Geometry: final body of the model. Coordinates: model frame, mm. Face numbers are marked on the shaded views. A direction names the side the tool comes from. Give positions to 0.01 mm unless a question says otherwise; leave off trailing zeros. Write each loop counter-clockwise with the first axis right and the second up, starting at its lowest first coordinate (ties: lowest second). Pieces come first, ordered by that corner, then holes.
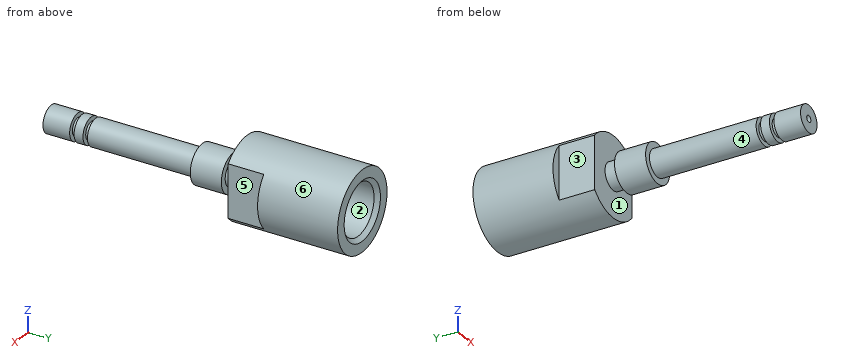
```python
from build123d import *

# Parameters (mm, degrees)
SKETCH17_R                    = 1.5
CUT_EXTRUDE1_DEPTH            = 65
G1_4_TAPPED_HOLE1_D           = 11.445
G1_4_TAPPED_HOLE1_DEPTH       = 22
G1_4_TAPPED_HOLE1_CSINK_D     = 13.207
G1_4_TAPPED_HOLE1_CSINK_ANGLE = 90
G1_4_TAPPED_HOLE1_TIP         = 3.438424892
SKETCH18_W                    = 13.595594723
SKETCH18_H                    = 16.071338344
CUT_EXTRUDE2_DEPTH            = 8


with BuildPart() as part:
    # Sketch1 → Revolve1 (revolve)
    with BuildSketch(Plane.XY):
        Polygon((-0.75, 0), (-0.75, 70), (-9, 70), (-9, 44), (-3, 44), (-3, 41), (-4.396039606, 41), (-4.396039606, 34), (-3, 34), (-3, 10), (-2, 10), (-2, 9), (-3, 9), (-3, 7), (-2, 7), (-2, 6), (-3, 6), (-3, 0), align=None)
    revolve(axis=Axis((0, 0, 0), (0, 1, 0)))

    # Sketch17 → Cut-Extrude1 (cut)
    with BuildSketch(Plane(origin=(0, 70, 0), x_dir=(1, 0, 0), z_dir=(0, 1, 0))):
        Circle(SKETCH17_R)
    extrude(amount=-CUT_EXTRUDE1_DEPTH, mode=Mode.SUBTRACT)

    # G1/4 Tapped Hole1
    with Locations(Plane(origin=(0, 70, 0), x_dir=(1, 0, 0), z_dir=(0, 1, 0))):
        with Locations((0, 0)):
            CounterSinkHole(G1_4_TAPPED_HOLE1_D / 2, G1_4_TAPPED_HOLE1_CSINK_D / 2, depth=G1_4_TAPPED_HOLE1_DEPTH, counter_sink_angle=G1_4_TAPPED_HOLE1_CSINK_ANGLE)
            with Locations((0, 0, -(G1_4_TAPPED_HOLE1_DEPTH + G1_4_TAPPED_HOLE1_TIP / 2))):  # 118° drill point
                Cone(0, G1_4_TAPPED_HOLE1_D / 2, G1_4_TAPPED_HOLE1_TIP, mode=Mode.SUBTRACT)

    # Sketch18 → Cut-Extrude2 (cut)
    with BuildSketch(Plane.XZ.offset(-44)):
        with Locations((-13.547797362, 0)):
            Rectangle(SKETCH18_W, SKETCH18_H)
        with Locations((13.547797362, 0)):
            Rectangle(SKETCH18_W, SKETCH18_H)
    extrude(amount=-CUT_EXTRUDE2_DEPTH, mode=Mode.SUBTRACT)


solid = part.part
```
Item 1: Line query: L1, parallel to Z at x = 0, y = 58; L2, parallel to Z at x = 0, y = 22.5; L3, parallel to Y at x = 7.25, z = -2.75. Output: solid intervals per line, ascending.
Found:
L1: z = -9 to -5.72, 5.72 to 9
L2: z = -3 to -1.5, 1.5 to 3
L3: y = 52 to 70
Item 2: Section A-A, the plane y = 40. Return the cut outline in (x, z).
Found:
outline: circle Ø8.79 at (0, 0); hole circle Ø3 at (0, 0)
Item 3: Section B-B, the plane x = 7.5. Return the cut outline in (y, z).
Found:
outline: (52, -4.97) - (70, -4.97) - (70, 4.97) - (52, 4.97) - close
Item 4: Pin query (flat end, axial travel): pin 1 Ø5 at (x, z) = (-0.5, -0.5) entering from -Y; pin 2 Ø3 at (x, z) = (0.5, 1) entering from +Y; pin 3 Ø6.5 at (y, z) = (46.5, -2) entering from +X; pin 4 Ø1 at (x, z) = (1, -2.5) entering from +Y. Return the tip coordinate at first contact, or that it passes through.
Found:
pin 1: stops at y = 0
pin 2: stops at y = 46.13
pin 3: stops at x = 6.75
pin 4: stops at y = 46.48
Item 5: Reachability of the marked faces 4, 5 and 6 from +Z, -Z, +X, -X, +Y, -Y: full face, straight path, thin tool, end or side. Return the list, or none.
Found:
face 4: -Y
face 5: +Z, -Z, +X, -Y
face 6: +Y, -Y
Item 6: Pull-direction query (X, two-part tool) for the marked faces 1, 2 and 3; classes: +X half, -X half, draft (parallel to the pull), parting line (faces both ways), or undercut.
Found:
face 1: draft
face 2: undercut
face 3: -X half
